from build123d import *

# Parameters (mm, degrees)
SKETCH1_W                = 20
SKETCH1_H                = 15
BOSS_EXTRUDE1_DEPTH      = 15
SKETCH2_R                = 2
BOSS_EXTRUDE2_DEPTH      = 5
BOSS_EXTRUDE3_DEPTH      = 15
BOSS_EXTRUDE3_DEPTH_BACK = 12.5
SKETCH4_R                = 1.5
CUT_EXTRUDE1_DEPTH       = 6
SKETCH4_3_R              = 2.5
SKETCH4_3_R_2            = 1.5
CUT_EXTRUDE2_DEPTH       = 3


with BuildPart() as part:
    # Sketch1 → Boss-Extrude1 (new body)
    with BuildSketch(Plane(origin=(0, 0, 0), x_dir=(0, 0, -1), z_dir=(1, 0, 0))):
        Rectangle(SKETCH1_W, SKETCH1_H)
    extrude(amount=BOSS_EXTRUDE1_DEPTH)

    # Sketch2 → Boss-Extrude2 (add)
    with BuildSketch(Plane.XY.offset(10)):
        with BuildLine():
            Line((15, -7.5), (10.015567122, -7.5))
            Line((10.015567122, -7.5), (10.015567122, -12.105755295))
            ThreePointArc((10.015567122, -12.105755295), (18.393285758, -16.172276101), (15, -7.5))
        make_face()
        with Locations((15, -12.5)):
            Circle(SKETCH2_R, mode=Mode.SUBTRACT)
    boss_extrude2 = extrude(amount=-BOSS_EXTRUDE2_DEPTH)

    # Mirror1: Boss-Extrude2 across plane
    add(boss_extrude2.mirror(Plane.XY))

    # Sketch3 → Boss-Extrude3 (add, two sides)
    with BuildSketch(Plane.XZ.offset(-7.5)) as boss_extrude3_sk:
        Polygon((-3, 10), (-3, 12.5), (-6, 12.5), (-6, -12.5), (-3, -12.5), (-3, -10), (0, -10), (0, 10), align=None)
    extrude(amount=BOSS_EXTRUDE3_DEPTH)
    extrude(boss_extrude3_sk.sketch, amount=-BOSS_EXTRUDE3_DEPTH_BACK)

    # Sketch4 → Cut-Extrude1 (cut)
    with BuildSketch(Plane(origin=(0, 0, 0), x_dir=(0, 0, -1), z_dir=(1, 0, 0))):
        with Locations((0, 13.75)):
            Circle(SKETCH4_R)
    extrude(amount=-CUT_EXTRUDE1_DEPTH, mode=Mode.SUBTRACT)

    # Sketch4<3> → Cut-Extrude2 (cut)
    with BuildSketch(Plane(origin=(0, 0, 0), x_dir=(0, 0, -1), z_dir=(1, 0, 0))):
        with Locations((0, 13.75)):
            Circle(SKETCH4_3_R)
        with Locations((0, 13.75)):
            Circle(SKETCH4_3_R_2, mode=Mode.SUBTRACT)
    extrude(amount=-CUT_EXTRUDE2_DEPTH, mode=Mode.SUBTRACT)


solid = part.part
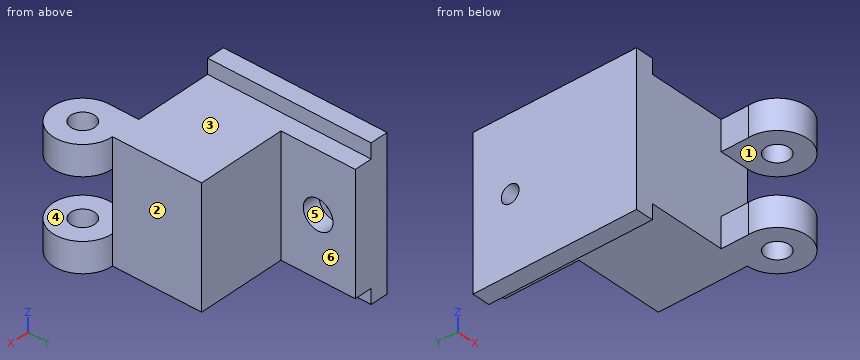
Here's how the part is built. I have some questions about the finished solid (model axes, mm). Face numbers are marked on the shaded views. A direction names the side the tool comes from. Coordinates: 2 decimals unless noted, no trailing zeros. Loops run counter-clockwise (first coordinate to the right, second up) from the corner with the lowest first, then second, coordinate; pieces in that order, holes last.
1. For P1, Ø8, axis at y = 13.75, z = 0, coming from the +X side; P2, Ø3, axis at x = -0.5, z = -8.5, coming from the -Y side; P3, Ø5, axis at x = 1.5, y = 0.5, coming from the -Z side, each with a flat end and sliding along its axis, tell me the tip position at first contact or that it passes through.
2. Imagine slicing it at A-A, the plane y = 13.75. Please give me the cut outline in (x, z), and give its area (3 significant figures).
3. If we mould it in two halves opening along Z, with no side actions, what happens to the marked faces 1, 2 and 3? For each: pulls with the +Z half, pulls with the -Z half, needs draft (parallel to the pull), parting line crosses it, or undercut.
4. Imagine slicing it at C-C, the plane z = 9.5. Please give me the cut outline in (x, y), and give its area (3 significant figures).
5. Imagine slicing it at B-B, the plane z = 0. Please give me the cut outline in (x, y), and give its area (3 significant figures).
6. Imagine slicing it at D-D, the plane x = -4.25. Please give me the cut outline in (y, z), and give its area (3 significant figures).
7. I need wall thicknesses on L1, parallel to Y at x = -0.9, z = 0; L2, parallel to Z at x = 13.5, y = -9; L3, parallel to X at y = 9.5, z = -9.5. Which ranges of each line are inside material? Lowest first, please.
8. For the marked faces 4, 5 and 6, which set-ups out of +Z, -Z, +X, -X, +Y, -Y let a thin tool reach every point of the face, with its end or its side?
Taken from the geometry:
1. P1: stops at x = 0
1. P2: stops at y = -7.5
1. P3: stops at z = -10
2. outline: (-6, -12.5) - (-3, -12.5) - (-3, -10) - (0, -10) - (0, -2.5) - (-3, -2.5) - (-3, -1.5) - (-6, -1.5) - close; (-6, 1.5) - (-3, 1.5) - (-3, 2.5) - (0, 2.5) - (0, 10) - (-3, 10) - (-3, 12.5) - (-6, 12.5) - close
2. area: 111 mm2
3. face 1: undercut
3. face 2: needs draft
3. face 3: pulls with the +Z half
4. outline: (-6, -7.5) - (10.02, -7.5) - (10.02, -12.11) arc R5 ccw (long way) to (15, -7.5) - (15, 7.5) - (0, 7.5) - (0, 20) - (-6, 20) - close; hole circle Ø4 at (15, -12.5)
4. area: 461 mm2
5. outline: (-6, -7.5) - (15, -7.5) - (15, 7.5) - (0, 7.5) - (0, 11.25) - (-3, 11.25) - (-3, 12.25) - (-6, 12.25) - close; (-6, 15.25) - (-3, 15.25) - (-3, 16.25) - (0, 16.25) - (0, 20) - (-6, 20) - close
5. area: 366 mm2
6. outline: (-7.5, -12.5) - (20, -12.5) - (20, 12.5) - (-7.5, 12.5) - close; hole circle Ø3 at (13.75, 0)
6. area: 680 mm2
7. L1: y = -7.5 to 11.25, 16.25 to 20
7. L2: z = -10 to -5, 5 to 10
7. L3: x = -6 to 0
8. face 4: +X, -X, -Y
8. face 5: +X
8. face 6: +Z, -Z, +X, +Y
